```python
from build123d import *

# Parameters (mm, degrees)
F0_R      = 228.6
F1_DEPTH  = 2286
F3_DEPTH  = 38.1
F6_W      = 38.1
F6_H      = 38.1
F8_W      = 38.1
F8_H      = 38.1
F9_DEPTH  = 279.4
F10_W     = 571.5
F10_H     = 38.1
F11_DEPTH = 38.1
F12_W     = 424.9351322651
F12_H     = 38.1
F13_DEPTH = 546.101
F14_R     = 228.6
F15_DEPTH = 4572


with BuildPart() as f1:
    # F0 (on Top) → F1 (new body, symmetric)
    with BuildSketch(Plane.XY):
        Circle(F0_R)
    extrude(amount=F1_DEPTH, both=True)

    # F2 (on Top) → F3 (join)
    with BuildSketch(Plane.XY):
        with BuildLine():
            ThreePointArc((-226.949, 0), (-160.4771768835, 160.4771768835), (0, 226.949))
            Line((0, 226.949), (0, 230.124))
            ThreePointArc((0, 230.124), (-162.7222409138, 162.7222409138), (-230.124, 0))
            Line((-230.124, 0), (-226.949, 0))
        make_face()
    extrude(amount=F3_DEPTH)

    # F4: F1 across face


with BuildPart() as f1_1:
    add(f1.part)
    add(f1.part.mirror(Plane(origin=(0, 229.362, 19.05), x_dir=(0, 1, 0), z_dir=(1, 0, 0))))

    # F6 (on offset) → F7 (join, up to the next surface of F1)
    with BuildSketch(Plane.YZ.offset(609.6)):
        with Locations((19.05, 19.05)):
            Rectangle(F6_W, F6_H)
    extrude(until=Until.NEXT, dir=(-1, 0, 0))

    # F8 (on face) → F9 (join)
    with BuildSketch(Plane(origin=(0, 38.1, 0), x_dir=(-1, 0, 0), z_dir=(0, 1, 0))):
        with Locations((-590.55, 19.05)):
            Rectangle(F8_W, F8_H)
        with Locations((-245.9981116379, 19.05)):
            Rectangle(F8_W, F8_H)
    extrude(amount=F9_DEPTH)

    # F10 (on face) → F11 (join)
    with BuildSketch(Plane(origin=(0, 317.5, 0), x_dir=(-1, 0, 0), z_dir=(0, 1, 0))):
        with Locations((-285.75, 19.05)):
            Rectangle(F10_W, F10_H)
    extrude(amount=-F11_DEPTH)

    # F12 (on face) → F13 (cut, through all)
    with BuildSketch(Plane(origin=(0, 317.5, 0), x_dir=(-1, 0, 0), z_dir=(0, 1, 0))):
        with Locations((212.4675661325, 19.05)):
            Rectangle(F12_W, F12_H)
    extrude(amount=-F13_DEPTH, mode=Mode.SUBTRACT)

    # F14 (on face) → F15 (cut)
    with BuildSketch(Plane.XY.offset(2286)):
        Circle(F14_R)
    extrude(amount=-F15_DEPTH, mode=Mode.SUBTRACT)

    # F16: F1 across face


with BuildPart() as f1_2:
    add(f1_1.part)
    add(f1_1.part.mirror(Plane(origin=(0, 298.45, 19.05), x_dir=(0, -1, 0), z_dir=(-1, 0, 0))))


solid = f1_2.part
```
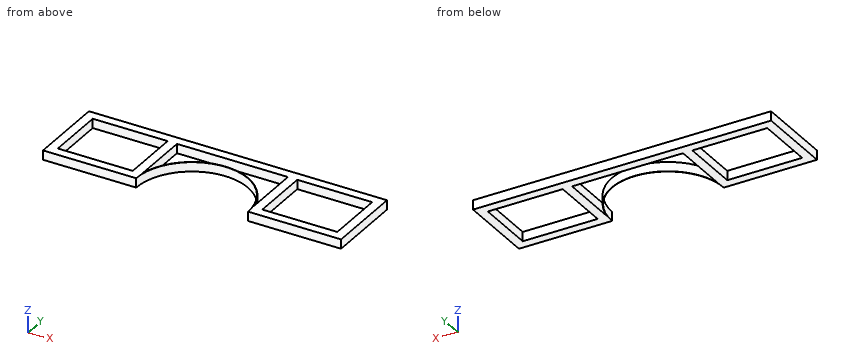
Input: part model. Units: mm. Frame: model coordinates. Give positions to 0.01 mm unless a question says otherwise; leave off trailing zeros. Order: outer loops, then holes, each group sorted by start corner. A loop starts at its lowest first (then second) coordinate and runs counter-clockwise, first axis right, second up. Notation, with made-up numbers: M -16.75,23 L 20.25,23 A22 ccw 20.25,43 Z; hole C 69,77 d3. An arc over 180 degrees is marked long. Return JSON: item names as keys, results as strings.
1) Contact query for a flat-ended pin moving along its axis: pin 1 (12 mm diameter, centred on x = -116.5, z = 19, fed in from -Y). Output: stop coordinate, or through.
Taken from the geometry:
{"pin 1": "stops at y = 193.01"}
2) Section query C-C on y = 152. Output: boundary loops of the cut face in (x, z), and give its area (3 significant figures).
Taken from the geometry:
{"outline": "M -609.6,0 L -571.5,0 L -571.5,38.1 L -609.6,38.1 Z; M -265.05,0 L -226.95,0 L -226.95,38.1 L -265.05,38.1 Z; M -172.78,0 L -170.75,0 L -170.75,38.1 L -172.78,38.1 Z; M 170.75,0 L 172.78,0 L 172.78,38.1 L 170.75,38.1 Z; M 226.95,0 L 265.05,0 L 265.05,38.1 L 226.95,38.1 Z; M 571.5,0 L 609.6,0 L 609.6,38.1 L 571.5,38.1 Z", "area": "5,960 mm2"}
3) Section query D-D on y = 102.5. Output: boundary loops of the cut face in (x, z), and give its area (3 significant figures).
Taken from the geometry:
{"outline": "M -609.6,0 L -571.5,0 L -571.5,38.1 L -609.6,38.1 Z; M -265.05,0 L -226.95,0 L -226.95,38.1 L -265.05,38.1 Z; M -206.04,0 L -204.33,0 L -204.33,38.1 L -206.04,38.1 Z; M 204.33,0 L 206.04,0 L 206.04,38.1 L 204.33,38.1 Z; M 226.95,0 L 265.05,0 L 265.05,38.1 L 226.95,38.1 Z; M 571.5,0 L 609.6,0 L 609.6,38.1 L 571.5,38.1 Z", "area": "5,940 mm2"}
4) Section query A-A on x = 0. Output: boundary loops of the cut face in (y, z), and give its area (3 significant figures).
Taken from the geometry:
{"outline": "M 228.6,0 L 230.12,0 L 230.12,38.1 L 228.6,38.1 Z; M 279.4,0 L 317.5,0 L 317.5,38.1 L 279.4,38.1 Z", "area": "1,510 mm2"}
5) Line query: L1, parallel to X at y = 249, z = 22.5; L2, parallel to Y at x = 543, z = 23; L3, parallel to Y at x = 7.5, z = 8. Output: solid intervals per line, ascending. Write a range as [from, to].
Taken from the geometry:
{"L1": "x = [-609.6, -571.5], [-265.05, -226.95], [226.95, 265.05], [571.5, 609.6]", "L2": "y = [0, 38.1], [279.4, 317.5]", "L3": "y = [228.48, 230], [279.4, 317.5]"}
6) Section query B-B on z = 10. Output: boundary loops of the cut face in (x, y).
Taken from the geometry:
{"outline": "M -609.6,0 L -228.6,0 A228.6 cw 228.6,0 L 609.6,0 L 609.6,317.5 L -609.6,317.5 Z; hole M -571.5,38.1 L -265.05,38.1 L -265.05,279.4 L -571.5,279.4 Z; hole M -226.95,38.1 A230.12 cw 226.95,38.1 L 226.95,279.4 L -226.95,279.4 Z; hole M 265.05,38.1 L 571.5,38.1 L 571.5,279.4 L 265.05,279.4 Z"}
